Could you check a few things on this drawing? It's one solid part, dimensions in mm from its lowest x, y, z. A direction names the side the tool comes from. Round coordinates to 2 decimals unless told otherwise and drop trailing zeros. Write each loop counter-clockwise with the first axis right and the second up, starting at its lowest first coordinate (ties: lowest second). Pieces come first, ordered by that corner, then holes. Notation, with made-up numbers: (-36.5, 10) -> (-9.5, 10) arc R21 cw to (-9.5, 28) -> close; hole circle Ø8 at (84, -1.5). An arc over 180 degrees is marked (long way). Return JSON: item names as keys, results as strings.
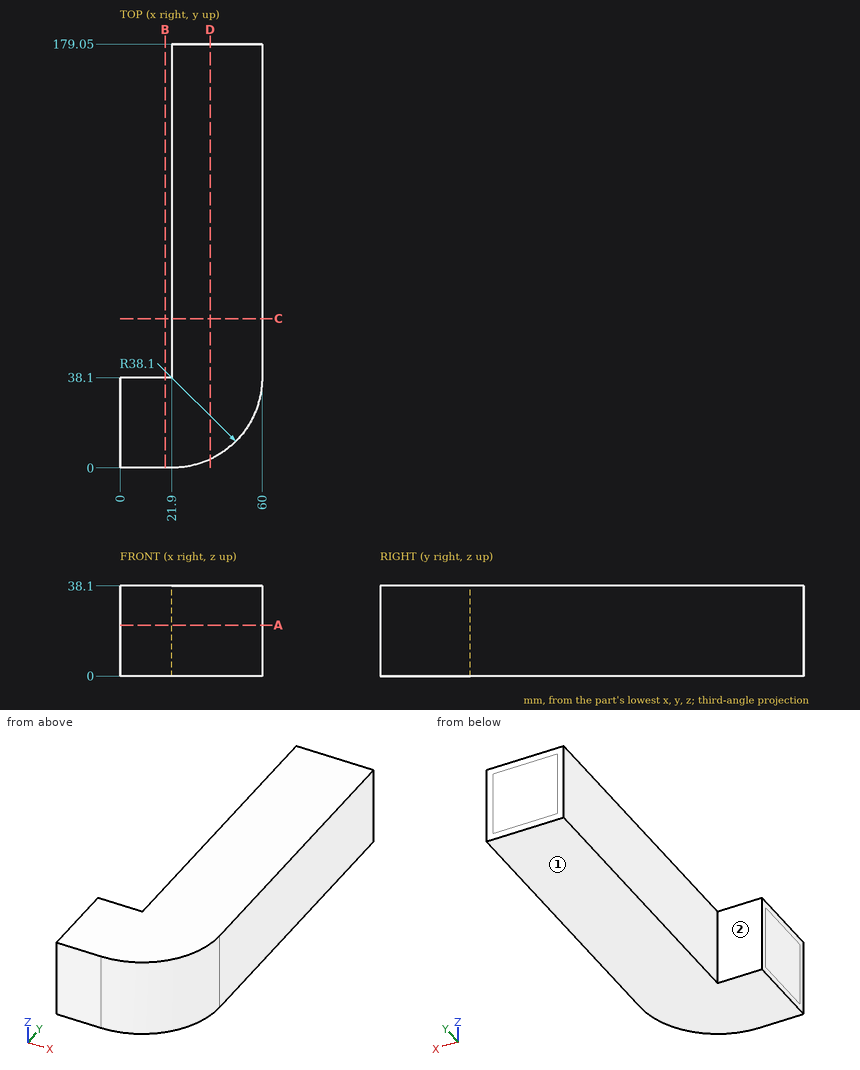
1) I want a section at D-D, the plane x = 38. Please give me the cut outline in (y, z) (3 decimals).
Return value:
{"outline": "(3.569, 0) -> (179.05, 0) -> (179.05, 38.1) -> (3.569, 38.1) -> close"}
2) I want a section at A-A, the plane z = 21.5. Please give me the cut outline in (x, y) (3 decimals).
Return value:
{"outline": "(0, 0) -> (21.9, 0) arc R38.1 ccw to (60, 38.1) -> (60, 179.05) -> (21.9, 179.05) -> (21.9, 38.1) -> (0, 38.1) -> close"}
3) Will these pins go through, and if not, where does the flat tip stop? pin 1 Ø10 at (y, z) = (130, 21) entering from -X; pin 2 Ø17.5 at (x, z) = (5.5, 17.5) entering from +Y.
Return value:
{"pin 1": "x = 21.9", "pin 2": "y = 38.1"}
4) For the marked faces 1 and 2, which set-ups out of +Z, -Z, +X, -X, +Y, -Y let a thin tool reach every point of the face, with its end or its side?
Return value:
{"face 1": "-Z, +X, -X, +Y, -Y", "face 2": "+Z, -Z, -X, +Y"}
5) If I drill on probe 1 along X at (y, z) = (120, 3.5); probe 2 along Y at (x, z) = (12, 28.5); probe 3 along X at (y, z) = (26, 9), over which ranges is the centre line in solid material (lowest first)? Write a range as [from, to].
Return value:
{"probe 1": "[21.9, 60]", "probe 2": "[0, 38.1]", "probe 3": "[0, 58.03]"}
6) I want a section at B-B, the plane x = 19. Please give me the cut outline in (y, z), and give its area (3 significant figures).
Return value:
{"outline": "(0, 0) -> (38.1, 0) -> (38.1, 38.1) -> (0, 38.1) -> close", "area": "1,450 mm²"}
7) I want a section at C-C, the plane y = 63. Please give me the cut outline in (x, z).
Return value:
{"outline": "(21.9, 0) -> (60, 0) -> (60, 38.1) -> (21.9, 38.1) -> close"}
